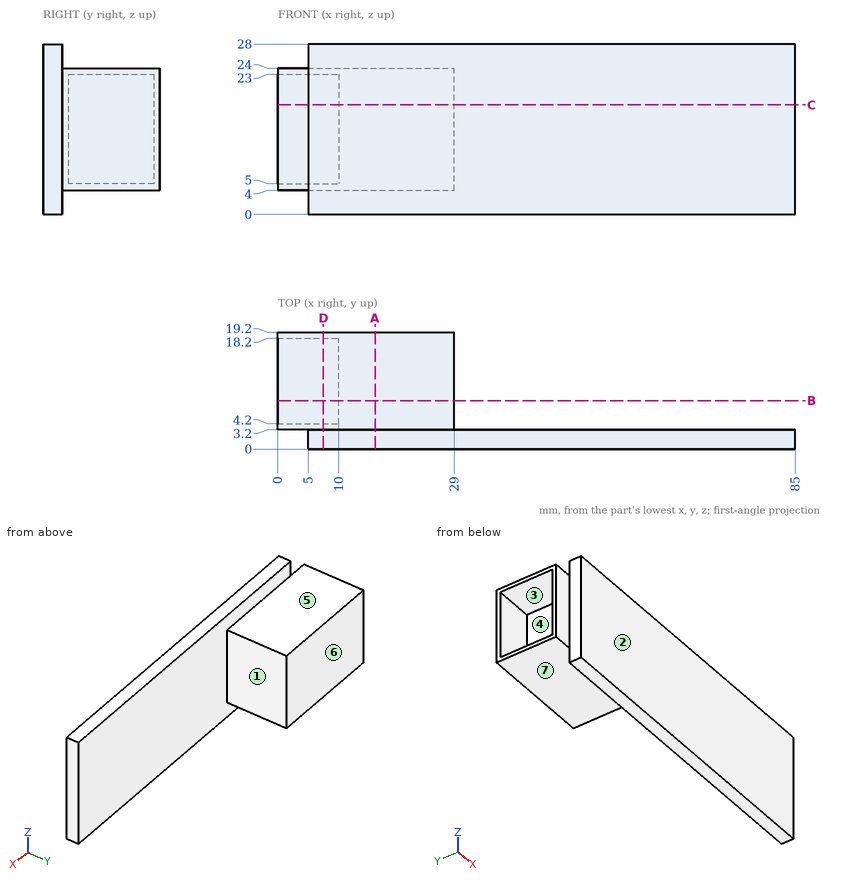
Can you work these out from the drawing? Everything is in mm from the part's minimum corner. A direction names the side the tool comes from. Round coordinates to 2 decimals unless told otherwise and drop trailing zeros. Write each loop counter-clockwise with the first axis right and the second up, starting at its lowest first coordinate (ties: lowest second). Pieces come first, ordered by that corner, then holes.
1. Suppose I cut it at B-B (y = 8). List the corners of the cut face in (x, z) for me.
2. Will these pins go through, and if not, where does the flat tip stop? pin 1 Ø4 at (y, z) = (14, 13) entering from -X; pin 2 Ø8 at (x, y) = (4.5, 13) entering from +Z; pin 3 Ø1.5 at (y, z) = (15, 14.5) entering from +X; pin 4 Ø10 at (x, y) = (42, 10.5) entering from +Z.
3. Suppose I cut it at A-A (x = 16). List the corners of the cut face in (y, z) for me.
4. If we mould it in two halves opening along Z, with no side actions, what happens to the marked faces 4, 5, 6 and 7? For each: released by +Z, released by -Z, zero draft, split by the parting line, or undercut.
5. Suppose I cut it at D-D (x = 7.5). List the corners of the cut face in (y, z) for me, and give its area (3 significant figures).
6. I need wall thicknesses on L1, parallel to Z at x = 7.5, y = 12.5; L2, parallel to X at y = 13.75, z = 9; L3, parallel to Y at x = 69.5, z = 24. Which ranges of each line are inside material? Lowest first, please.
7. Suppose I cut it at C-C (z = 18). List the corners of the cut face in (x, y) for me, and give its area (3 significant figures).
8. For the marked faces 1, 2 and 3, which set-ups out of +Z, -Z, +X, -X, +Y, -Y let a thin tool reach every point of the face, with its end or its side?
Answer sheet:
1. outline: (0, 4) - (29, 4) - (29, 24) - (0, 24) - (0, 23) - (10, 23) - (10, 5) - (0, 5) - close
2. pin 1: stops at x = 10
2. pin 2: stops at z = 24
2. pin 3: stops at x = 29
2. pin 4: passes through
3. outline: (0, 0) - (3.2, 0) - (3.2, 4) - (19.2, 4) - (19.2, 24) - (3.2, 24) - (3.2, 28) - (0, 28) - close
4. face 4: undercut
4. face 5: released by +Z
4. face 6: zero draft
4. face 7: released by -Z
5. outline: (0, 0) - (3.2, 0) - (3.2, 4) - (19.2, 4) - (19.2, 24) - (3.2, 24) - (3.2, 28) - (0, 28) - close; hole (4.2, 5) - (18.2, 5) - (18.2, 23) - (4.2, 23) - close
5. area: 158 mm2
6. L1: z = 4 to 5, 23 to 24
6. L2: x = 10 to 29
6. L3: y = 0 to 3.2
7. outline: (0, 3.2) - (5, 3.2) - (5, 0) - (85, 0) - (85, 3.2) - (29, 3.2) - (29, 19.2) - (0, 19.2) - (0, 18.2) - (10, 18.2) - (10, 4.2) - (0, 4.2) - close
7. area: 580 mm2
8. face 1: +Z, -Z, +X, +Y
8. face 2: +Z, -Z, +X, -X, -Y
8. face 3: -X
